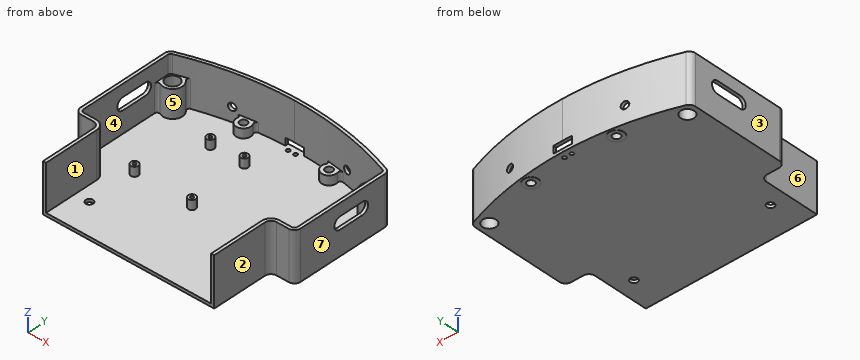
```python
from build123d import *

# Parameters (mm, degrees)
F1_DEPTH       = 40
F2_W           = 100
F2_H           = 200
F3_DEPTH       = 100
F4_R           = 5
F5_T           = -2.5
F6_R           = 3
F7_DEPTH       = 25
F8_R           = 8
F9_DEPTH       = 25
F10_R          = 5.5
F11_DEPTH      = 25
F12_R          = 3
F12_R_2        = 1.25
F13_DEPTH      = 10
F14_R          = 3
F15_DEPTH      = 150
F17_START      = -41.94633
F16_W          = 15
F16_H          = 6
F17_DEPTH      = 208.05367
F18_R          = 1.5
F19_DEPTH      = 12.5
F20_R          = 6
F21_DEPTH      = 0.2
F21_DEPTH_BACK = 10
F22_R          = 3
F23_DEPTH      = 12.5
F24_R          = 2
F26_DEPTH      = 150


with BuildPart() as f1:
    # F0 (on Top) → F1 (new body)
    with BuildSketch(Plane.XY):
        with BuildLine():
            Line((-90, 83.2380757938), (-90, -50))
            Line((-90, -50), (90, -50))
            Line((90, -50), (90, 83.2380757938))
            ThreePointArc((90, 83.2380757938), (45.7737973711, 95.7737973711), (0, 100))
            ThreePointArc((0, 100), (-45.7737973711, 95.7737973711), (-90, 83.2380757938))
        make_face()
    extrude(amount=F1_DEPTH)

    # F2 (on Top) → F3 (cut)
    with BuildSketch(Plane.XY):
        with Locations((-120, -100)):
            Rectangle(F2_W, F2_H)
        with Locations((120, -100)):
            Rectangle(F2_W, F2_H)
    extrude(amount=F3_DEPTH, mode=Mode.SUBTRACT)

    # F4
    f4_edges = [f1.edges().sort_by_distance(p)[0] for p in [
        (-90, 83.238076, 20),
        (90, 83.238076, 20),
        (90, 0, 20),
        (70, 0, 20),
        (-90, 0, 20),
        (-70, 0, 20),
    ]]
    fillet(f4_edges, radius=F4_R)

    # F5
    f5_openings = [f1.faces().sort_by_distance(p)[0] for p in [
        (0, 26.262097, 40),
        (0, -50, 20),
    ]]
    offset(amount=F5_T, openings=f5_openings)

    # F6 (on Top) → F7 (cut)
    with BuildSketch(Plane.XY):
        with Locations((-55.8614357137, -24.1385642863)):
            Circle(F6_R)
        with Locations((55.8614357137, -24.1385642863)):
            Circle(F6_R)
    extrude(amount=F7_DEPTH, mode=Mode.SUBTRACT)

    # F8 (on Top) → F9 (join)
    with BuildSketch(Plane.XY):
        with Locations((-81, 77)):
            Circle(F8_R)
        with Locations((81, 77)):
            Circle(F8_R)
    extrude(amount=F9_DEPTH)

    # F10 (on Top) → F11 (cut)
    with BuildSketch(Plane.XY):
        with Locations((-81, 77)):
            Circle(F10_R)
        with Locations((81, 77)):
            Circle(F10_R)
    extrude(amount=F11_DEPTH, mode=Mode.SUBTRACT)

    # F12 (on Top) → F13 (join)
    with BuildSketch(Plane.XY):
        with Locations((-55, 15)):
            Circle(F12_R)
        with Locations((-55, 15)):
            Circle(F12_R_2, mode=Mode.SUBTRACT)
        with Locations((-39.8, 65.8)):
            Circle(F12_R)
        with Locations((-39.8, 65.8)):
            Circle(F12_R_2, mode=Mode.SUBTRACT)
        with Locations((-11.9, 65.8)):
            Circle(F12_R)
        with Locations((-11.9, 65.8)):
            Circle(F12_R_2, mode=Mode.SUBTRACT)
        with Locations((-6.8, 13.7)):
            Circle(F12_R)
        with Locations((-6.8, 13.7)):
            Circle(F12_R_2, mode=Mode.SUBTRACT)
    extrude(amount=F13_DEPTH)

    # F14 (on Front) → F15 (cut, symmetric)
    with BuildSketch(Plane.XZ):
        with Locations((47, 14)):
            Circle(F14_R)
        with Locations((-47, 14)):
            Circle(F14_R)
    extrude(amount=F15_DEPTH, both=True, mode=Mode.SUBTRACT)

    # F16 (on Front) → F17 (cut)
    with BuildSketch(Plane.XZ.offset(F17_START)):
        with Locations((0, 5.5)):
            Rectangle(F16_W, F16_H)
    extrude(amount=-F17_DEPTH, mode=Mode.SUBTRACT)

    # F18 (on Top) → F19 (cut, symmetric)
    with BuildSketch(Plane.XY):
        with Locations((-3, 95)):
            Circle(F18_R)
        with Locations((3, 95)):
            Circle(F18_R)
    extrude(amount=F19_DEPTH, both=True, mode=Mode.SUBTRACT)

    # F20 (on Top) → F21 (join, two sides)
    with BuildSketch(Plane.XY) as f21_sk:
        with Locations((-35, 90)):
            Circle(F20_R)
        with Locations((35, 90)):
            Circle(F20_R)
    extrude(amount=-F21_DEPTH)
    extrude(f21_sk.sketch, amount=F21_DEPTH_BACK)

    # F22 (on face) → F23 (cut, symmetric)
    with BuildSketch(Plane(origin=(0, 0, 0), x_dir=(1, 0, 0), z_dir=(0, 0, -1))):
        with Locations((-35, -90)):
            Circle(F22_R)
        with Locations((35, -90)):
            Circle(F22_R)
    extrude(amount=F23_DEPTH, both=True, mode=Mode.SUBTRACT)

    # F24
    f24_edges = [f1.edges().sort_by_distance(p)[0] for p in [
        (-87.5, 72.33631, 13.75),
        (-78.687247, 84.658405, 13.75),
        (-32.339812, 95.378048, 6.25),
        (-39.085326, 94.394328, 6.25),
        (39.085326, 94.394328, 6.25),
        (32.339812, 95.378048, 6.25),
        (78.687247, 84.658405, 13.75),
        (87.5, 72.33631, 13.75),
    ]]
    fillet(f24_edges, radius=F24_R)

    # F25 (on Right) → F26 (cut, symmetric)
    with BuildSketch(Plane.YZ):
        with BuildLine():
            Line((40, 20), (40, 30))
            ThreePointArc((40, 30), (35, 25), (40, 20))
        make_face()
        with BuildLine():
            ThreePointArc((65, 25), (63.5355339059, 28.5355339059), (60, 30))
            Line((60, 30), (60, 20))
            ThreePointArc((60, 20), (63.5355339059, 21.4644660941), (65, 25))
        make_face()
        with BuildLine():
            Line((60, 30), (40, 30))
            ThreePointArc((40, 30), (43.5355339059, 28.5355339059), (45, 25))
            ThreePointArc((45, 25), (43.5355339059, 21.4644660941), (40, 20))
            Line((40, 20), (60, 20))
            ThreePointArc((60, 20), (55, 25), (60, 30))
        make_face()
        with BuildLine():
            ThreePointArc((45, 25), (43.5355339059, 28.5355339059), (40, 30))
            Line((40, 30), (40, 20))
            ThreePointArc((40, 20), (43.5355339059, 21.4644660941), (45, 25))
        make_face()
        with BuildLine():
            Line((60, 20), (60, 30))
            ThreePointArc((60, 30), (55, 25), (60, 20))
        make_face()
    extrude(amount=F26_DEPTH, both=True, mode=Mode.SUBTRACT)


solid = f1.part
```
The listing builds one solid part. Answer for the finished solid, in the listing's coordinates (mm). Face numbers are marked on the shaded views. A direction names the side the tool comes from. Give positions to 0.01 mm unless a question says otherwise; leave off trailing zeros. Order: outer loops, then holes, each group sorted by start corner. A loop starts at its lowest first (then second) coordinate and runs counter-clockwise, first axis right, second up. Notation, with made-up numbers: (26, 10.25) -> (30, 10.25) arc R11 ccw to (30, 24.25) -> close; hole circle Ø5 at (69.5, 15.25). An arc over 180 degrees is marked (long way). One line per item, written item: value.
1) Determine the mould class of the marked faces 5, 6 and 7 for opening direction X: pulls with the +X half, pulls with the -X half, needs draft (parallel to the pull), parting line crosses it, or undercut.
Reported:
face 5: undercut
face 6: pulls with the -X half
face 7: pulls with the +X half
2) Find section D-D, the plane x = 47. Determine the outline of the cut face in (y, z).
Reported:
outline: (-50, 0) -> (95.54, 0) -> (95.54, 11) -> (93, 11) -> (93, 2.5) -> (-50, 2.5) -> close; (93, 17) -> (95.54, 17) -> (95.54, 40) -> (93, 40) -> close
3) Find section B-B, the plane y = 24. Determine the outline of the cut face in (x, z), plus the area to 4 significant figures.
Reported:
outline: (-90, 0) -> (90, 0) -> (90, 40) -> (87.5, 40) -> (87.5, 2.5) -> (-87.5, 2.5) -> (-87.5, 40) -> (-90, 40) -> close
area: 637.5 mm^2
4) Find section A-A, the plane y = 54. Determine the outline of the cut face in (x, z), plus the area to 4 significant figures.
Reported:
outline: (-90, 0) -> (90, 0) -> (90, 20) -> (87.5, 20) -> (87.5, 2.5) -> (-87.5, 2.5) -> (-87.5, 20) -> (-90, 20) -> close; (-90, 30) -> (-87.5, 30) -> (-87.5, 40) -> (-90, 40) -> close; (87.5, 30) -> (90, 30) -> (90, 40) -> (87.5, 40) -> close
area: 587.5 mm^2
5) Find the intervals of material crossed by line 1 (Y direction, x = 81, z = 15.5); line 2 (X direction, y = 34.5, z = 29); line 3 (Y direction, x = -55, z = 5), in increasing order.
Reported:
line 1: y = 0 to 2.5, 69 to 71.5, 82.5 to 86.51
line 2: x = -90 to -87.5, 87.5 to 90
line 3: y = 12 to 13.75, 16.25 to 18, 91.31 to 93.87
6) Find section C-C, the plane z = 35. Determine the outline of the cut face in (x, y).
Reported:
outline: (-90, 5) arc R5 ccw to (-85, 0) -> (-75, 0) arc R5 cw to (-70, -5) -> (-70, -50) -> (-67.5, -50) -> (-67.5, -5) arc R7.5 ccw to (-75, 2.5) -> (-85, 2.5) arc R2.5 cw to (-87.5, 5) -> (-87.5, 79.78) arc R2.5 cw to (-85.87, 82.13) arc R247.5 cw to (85.87, 82.13) arc R2.5 cw to (87.5, 79.78) -> (87.5, 5) arc R2.5 cw to (85, 2.5) -> (75, 2.5) arc R7.5 ccw to (67.5, -5) -> (67.5, -50) -> (70, -50) -> (70, -5) arc R5 cw to (75, 0) -> (85, 0) arc R5 ccw to (90, 5) -> (90, 79.78) arc R5 ccw to (86.73, 84.47) arc R250 ccw to (-86.73, 84.47) arc R5 ccw to (-90, 79.78) -> close
7) Flat-ended cylindrical pins translate along their axes: P1, Ø8, axis at x = -80.5, z = 14, coming from the -Y side; P2, Ø1.8, axis at x = -5.5, y = 14, coming from the +Z side; P3, Ø2, axis at x = -38.5, y = 30.5, coming from the -Z side; P4, Ø3.5, axis at x = -47, z = 14, coming from the -Y side. Find the tip coordinate at first contact, or state that the pin passes through.
Reported:
P1: stops at y = 0
P2: stops at z = 10
P3: stops at z = 0
P4: passes through
8) A tool of negligible diameter and unlimited length cuts with its end or side. For the marked faces 1, 2, 3 and 4, from which of +Z, -Z, +X, -X, +Y, -Y can it reach the whole face along a straight path? Write none if from no direction.
Reported:
face 1: +Z, -Y
face 2: +Z, -Z, +X, -Y
face 3: +Z, -Z, -X, +Y, -Y
face 4: +Z
